Part print with two shaded views. Sizes in mm from the minimum x, y, z corner. A direction names the side the tool comes from. Coordinates: 2 decimals unless noted, no trailing zeros. Loops run counter-clockwise (first coordinate to the right, second up) from the corner with the lowest first, then second, coordinate; pieces in that order, holes last.
(1) Slice it at A-A (x = 35.5). Give the cut face in (y, z).
(2) Two-plate mould, pull along Z, no slides. Class the marked faces 3, 4 and 5: pulls with the +Z half, pulls with the -Z half, needs draft (parallel to the pull), parting line crosses it, or undercut.
(3) Flat gauge pins, fed straight in: P1, Ø6, axis at x = 23, z = 3, coming from the +Y side; P2, Ø1, axis at y = 7, z = 3.5, coming from the -X side. Where does each tip first touch, or does it go through?
(4) Wall check: L1, parallel to Y at x = 10, z = 7.5; L2, parallel to Y at x = 61, z = 5.5; L3, parallel to Y at x = 25, z = 3.5. Give the ranges that are in metal, low to high.
(5) Slice it at C-C (z = 1). Give the cut face in (x, y).
(6) Tool access for the marked faces 1 and 2: list every direction of +Z, -Z, +X, -X, +Y, -Y with a clear straight run to the whole face (end or side of a thin tool).
(7) Slice it at D-D (x = 61). Give the cut face in (y, z).
(8) Slice it at B-B (y = 6). Give the cut face in (x, z), and give its area (3 significant figures).
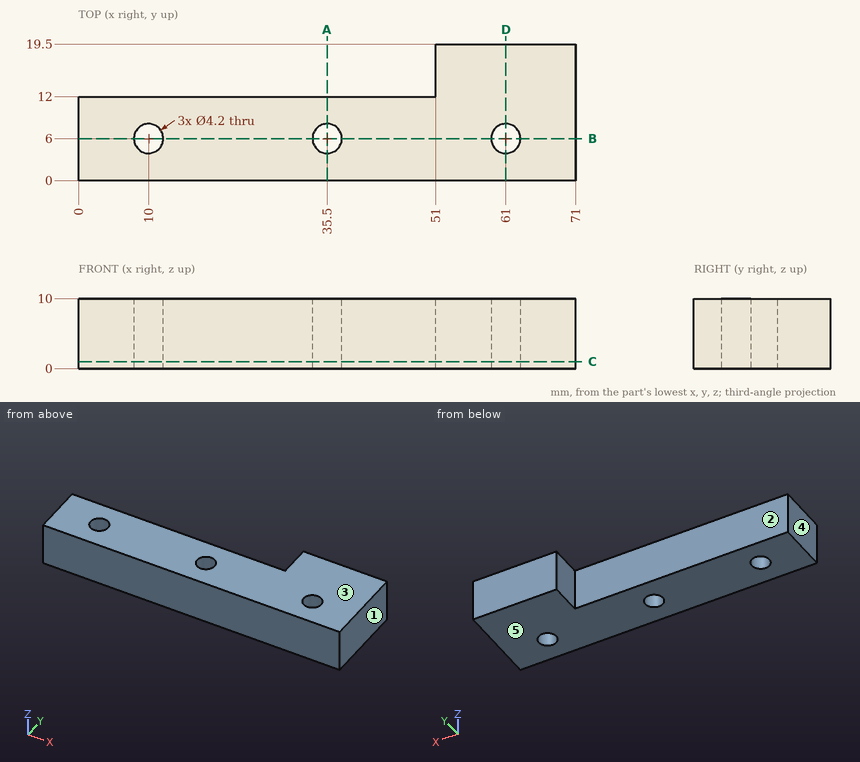
Response values:
1. outline: (0, 0) - (3.9, 0) - (3.9, 10) - (0, 10) - close; (8.1, 0) - (12, 0) - (12, 10) - (8.1, 10) - close
2. face 3: pulls with the +Z half
2. face 4: needs draft
2. face 5: pulls with the -Z half
3. P1: stops at y = 12
3. P2: stops at x = 0
4. L1: y = 0 to 3.9, 8.1 to 12
4. L2: y = 0 to 3.9, 8.1 to 19.5
4. L3: y = 0 to 12
5. outline: (0, 0) - (71, 0) - (71, 19.5) - (51, 19.5) - (51, 12) - (0, 12) - close; hole circle Ø4.2 at (10, 6); hole circle Ø4.2 at (35.5, 6); hole circle Ø4.2 at (61, 6)
6. face 1: +Z, -Z, +X, +Y, -Y
6. face 2: +Z, -Z, -X, +Y
7. outline: (0, 0) - (3.9, 0) - (3.9, 10) - (0, 10) - close; (8.1, 0) - (19.5, 0) - (19.5, 10) - (8.1, 10) - close
8. outline: (0, 0) - (7.9, 0) - (7.9, 10) - (0, 10) - close; (12.1, 0) - (33.4, 0) - (33.4, 10) - (12.1, 10) - close; (37.6, 0) - (58.9, 0) - (58.9, 10) - (37.6, 10) - close; (63.1, 0) - (71, 0) - (71, 10) - (63.1, 10) - close
8. area: 584 mm2
